The listing builds one solid part. Answer for the finished solid, in the listing's coordinates (mm). A direction names the side the tool comes from. Give positions to 0.01 mm unless a question says otherwise; leave off trailing zeros. Loops run counter-clockwise (first coordinate to the right, second up) from the corner with the lowest first, then second, coordinate; pieces in that order, holes last. Notation, with made-up numbers: M 76,52.25 L 109,52.25 A29 ccw 109,91.25 Z; hole C -22.75,82.5 d5. An arc over 180 degrees is marked long. Use one line per item in the form item = value. Start each with the question number.
1. For faces 1 (the face through (5.5, 34.8, -5)), 2 (the face through (5.07, 35.49, -4.28)), determine the directions among +Z, -Z, +X, -X, +Y, -Y from which every point of the face is accessible in a straight line to the end or side of a thin tool.
2. Straight lines are drawn through the part: line 1 (X direction, y = 23, z = -15.5) (3 decimals); line 2 (X direction, y = 27, z = -23); line 3 (Z direction, x = 1.5, y = 23.5). For each, find the intervals that lie inside material, in ascending order. Write a range as from..to.
3. The mould has two halves that part along X. Classify faces 3 (the face through (2, 12, 0)), 4 (the face through (5.5, 34.8, -25)), 5 (the face through (5, 20, -15)): released by +X, released by -X, zero draft, split by the parting line, or undercut.
4. Each of these flat-tipped pins is pushed along its axis until it touches: pin 1 Ø5 at (x, y) = (6.5, 34.5) entering from -Z; pin 2 Ø2 at (y, z) = (22.5, -8.5) entering from -X; pin 3 Ø6 at (y, z) = (28.5, -21.5) entering from -X. Where does it stop, or does it pass through?
5. The part is cut by section A-A (y = 9.5). Write down the section's boundary in (x, z), and give its area (3 significant figures).
6. The part is cut by section C-C (x = 3). Write down the section's boundary in (y, z), and give its area (3 significant figures).
7. The part is cut by section B-B (z = -2). Write down the section's boundary in (x, y).
from build123d import *

# Parameters (mm, degrees)
SKETCH1_W           = 10
SKETCH1_H           = 30
BOSS_EXTRUDE1_DEPTH = 40
FILLET1_R           = 15
CUT_EXTRUDE1_DEPTH  = 40
SHELL2_T            = -1


with BuildPart() as part:
    # Sketch1 → Boss-Extrude1 (new body)
    with BuildSketch(Plane(origin=(0, 0, 0), x_dir=(1, 0, 0), z_dir=(0, 1, 0))):
        with Locations((5, 15)):
            Rectangle(SKETCH1_W, SKETCH1_H)
    extrude(amount=BOSS_EXTRUDE1_DEPTH)

    # Fillet1
    fillet1_edges = [part.edges().sort_by_distance(p)[0] for p in [
        (5, 40, -30),
        (5, 40, 0),
    ]]
    fillet(fillet1_edges, radius=FILLET1_R - 0.0001)  # a hair under: the kernel refuses the full size

    # Sketch2 → Cut-Extrude1 (cut)
    with BuildSketch(Plane.XZ):
        with BuildLine():
            Line((10, 0), (5, 0))
            ThreePointArc((5, 0), (8.717082451, -7.09430585), (10, -15))
            Line((10, -15), (10, 0))
        make_face()
        with BuildLine():
            Line((10, -30), (10, -15))
            ThreePointArc((10, -15), (8.717082451, -22.90569415), (5, -30))
            Line((5, -30), (10, -30))
        make_face()
        with BuildLine():
            ThreePointArc((0, 0), (5, -15), (0, -30))
            Line((0, -30), (0, 0))
        make_face()
    extrude(amount=-CUT_EXTRUDE1_DEPTH, mode=Mode.SUBTRACT)

    # Shell2
    shell2_openings = [part.faces().sort_by_distance(p)[0] for p in [
        (5.9062731, 0, -15),
    ]]
    offset(amount=SHELL2_T, openings=shell2_openings)


solid = part.part
Derived:
q1.face_1 = -Y
q1.face_2 = +Z, +X, -X, +Y
q2.line_1 = 4.995..5.995, 8.995..9.995
q2.line_2 = 3.69..4.74, 7.63..8.69
q2.line_3 = -30..-27.76, -2.24..0
q3.face_3 = zero draft
q3.face_4 = undercut
q3.face_5 = released by -X
q4.pin_1 = -28.26
q4.pin_2 = 3.85
q4.pin_3 = 3.12
q5.outline = M 0,-30 L 5,-30 A25 ccw 5,0 L 0,0 A25 cw Z; hole M 1.91,-29 L 4.49,-29 A24 ccw 4.49,-1 L 1.91,-1 A26 cw Z
q5.area = 69.4 mm2
q6.outline = M 0,-30 L 25,-30 A15 ccw 36.36,-24.8 L 0,-24.8 L 0,-27.12 L 32,-27.12 A14 cw 25,-29 L 0,-29 Z; M 0,-5.2 L 36.36,-5.2 A15 ccw 25,0 L 0,0 L 0,-1 L 25,-1 A14 cw 32,-2.88 L 0,-2.88 Z
q6.area = 231 mm2
q7.outline = M 1.35,0 L 2.52,0 L 2.52,30.2 L 5.17,30.2 L 5.17,0 L 6.35,0 L 6.35,32.48 L 1.35,32.48 Z
